The model under review builds one solid part; all positions refer to its coordinate system, in mm. Face numbers are marked on the shaded views. A direction names the side the tool comes from. Coordinates: 2 decimals unless noted, no trailing zeros. Order: outer loops, then holes, each group sorted by start corner. A loop starts at its lowest first (then second) coordinate and runs counter-clockwise, first axis right, second up. Notation, with made-up numbers: M 6,74.5 L 13,74.5 A9 cw 13,79.5 Z; hole C -21.75,9.25 d6. An arc over 180 degrees is marked long. One line per item, written item: value.
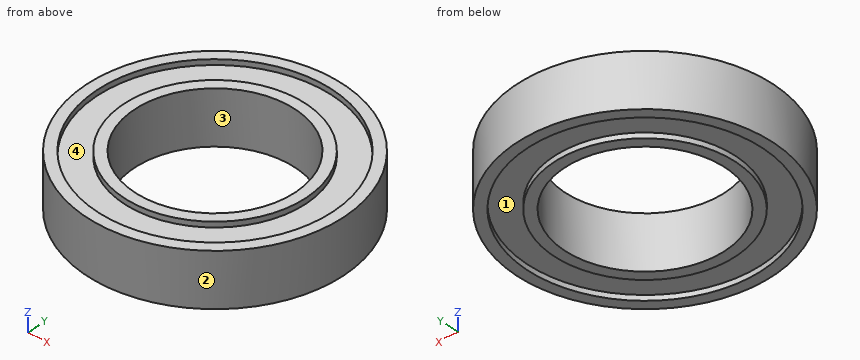
Autodesk Inventor part; units mm, degrees
ref_plane "YZ Plane" through (0, 0, 0) normal (1, 0, 0) x (0, 1, 0)
ref_plane "XZ Plane" through (0, 0, 0) normal (0, 1, 0) x (-1, 0, 0)
ref_plane "XY Plane" through (0, 0, 0) normal (0, 0, 1) x (1, 0, 0)
sketch "スケッチ1" plane through (0, 0, 0) normal (0, 0, 1) x (1, 0, 0)
  circle A0 centre (0, 0) radius 7.5
  circle A1 centre (0, 0) radius 12
  dimension "d0" = 15
  dimension "d1" = 24
extrude "押し出し1" add sketch "スケッチ1" along normal blind 5
sketch "スケッチ2" plane through (0, 0, 5) normal (0, 0, 1) x (1, 0, 0)
  circle A0 centre (0, 0) radius 7.5
  circle A1 centre (0, 0) radius 12
  circle A2 centre (0, 0) radius 8.5
  circle A3 centre (0, 0) radius 11
  dimension "d4" = 1
  dimension "d5" = 1
extrude "押し出し2" cut sketch "スケッチ2" against normal blind 0.5 contours A3
sketch "スケッチ3" plane through (0, 0, 0) normal (0, 0, -1) x (-1, 0, 0)
  circle A0 centre (0, 0) radius 11
  circle A1 centre (0, 0) radius 8.5
extrude "押し出し3" cut sketch "スケッチ3" against normal blind 0.5
properties part number "ベアリングd15-D24-B5" material "鋼、炭素鋼"
(1) For L1, parallel to Y at x = 0, z = 0.1; L2, parallel to Y at x = 0, z = 3.2; L3, parallel to Y at x = 5, z = 4.6, list the stretches that pass through material, from the lowest coordinate up.
Geometry results:
L1: y = -12 to -11, -8.5 to -7.5, 7.5 to 8.5, 11 to 12
L2: y = -12 to -7.5, 7.5 to 12
L3: y = -10.91 to -9.8, -6.87 to -5.59, 5.59 to 6.87, 9.8 to 10.91
(2) Tool access review of the marked faces 3 and 4: name each direction out of +Z, -Z, +X, -X, +Y, -Y from which nothing blocks a thin tool from reaching the whole face with its end or side.
Geometry results:
face 3: +Z, -Z
face 4: +Z
(3) We need section C-C, the plane z = 1.2. State the section outline as (x, y) points, plus the area to 3 significant figures.
Geometry results:
outline: C 0,0 d24; hole C 0,0 d15
area: 276 mm2
(4) We need section D-D, the plane y = -10.5. State the section outline as (x, z) points.
Geometry results:
outline: M -5.81,0 L -3.28,0 L -3.28,0.5 L 3.28,0.5 L 3.28,0 L 5.81,0 L 5.81,5 L 3.28,5 L 3.28,4.5 L -3.28,4.5 L -3.28,5 L -5.81,5 Z
(5) We need section A-A, the plane x = 0. State the section outline as (y, z) points.
Geometry results:
outline: M -12,0 L -11,0 L -11,0.5 L -8.5,0.5 L -8.5,0 L -7.5,0 L -7.5,5 L -8.5,5 L -8.5,4.5 L -11,4.5 L -11,5 L -12,5 Z; M 7.5,0 L 8.5,0 L 8.5,0.5 L 11,0.5 L 11,0 L 12,0 L 12,5 L 11,5 L 11,4.5 L 8.5,4.5 L 8.5,5 L 7.5,5 Z
(6) Mouldability with a two-part tool opening along X and no side actions: class the marked faces 1 and 2 as +X half, -X half, draft (parallel to the pull), parting line (faces both ways), or undercut.
Geometry results:
face 1: undercut
face 2: parting line
